Here's how the part is built. I have some questions about the finished solid (model axes, mm). Face numbers are marked on the shaded views. A direction names the side the tool comes from. Coordinates: 2 decimals unless noted, no trailing zeros. Write each loop counter-clockwise with the first axis right and the second up, starting at its lowest first coordinate (ties: lowest second). Pieces come first, ordered by that corner, then holes.
Item 1: I want a section at A-A (y = 6.1). Please give me the cut outline in (x, z) (3 decimals), and give its area (3 significant figures).
Item 2: For the marked faces 1 and 2, which set-ups out of +Z, -Z, +X, -X, +Y, -Y let a thin tool reach every point of the face, with its end or its side?
Item 3: If we mould it in two halves opening along Y, with no side actions, what happens to the marked faces 3, 4, 5 and 6? For each: pulls with the +Y half, pulls with the -Y half, needs draft (parallel to the pull), parting line crosses it, or undercut.
Item 4: I want a section at C-C (x = 3.5). Please give me the cut outline in (y, z) (3 decimals).
Item 5: I want a section at B-B (z = 8.75). Please give me the cut outline in (x, y) (3 decimals).
Item 6: I'm going to push flat-ended pins straight in: P1, Ø1.5, axis at x = 4.5, z = 7, coming from the -Y side; P2, Ø1.1, axis at y = 6, z = 8.5, coming from the -X side; P3, Ø1.1, axis at y = 7, z = 7, coming from the +X side. Where does each tip first touch, or does it pass through?
Item 7: I want a section at D-D (y = 10.5). Please give me the cut outline in (x, z), and give its area (3 significant figures).
Item 8: Please list where these lines run through material, in increasing order: line 1 (Z direction, x = 7, y = 10.25); line 2 (Y direction, x = 4.75, z = 6.25) (3 decimals); line 3 (Y direction, x = 0.75, z = 1.25).
Autodesk Inventor part; units mm, degrees
ref_plane "Work Plane1" through (0, 0, 5) normal (0, 0, 1) x (1, 0, 0)
ref_plane "YZ Plane" through (0, 0, 0) normal (1, 0, 0) x (0, 1, 0)
ref_plane "XZ Plane" through (0, 0, 0) normal (0, 1, 0) x (-1, 0, 0)
sketch "Sketch1" plane through (0, 0, 0) normal (0, 0, 1) x (1, 0, 0)
  line L0 (14.6962, 12.74) -> (14.6962, 0) construction
  line L1 (10.61, 12.2) -> (1.53, 12.2)
  arc A0 (1.53, 12.2) -> (0, 10.67) centre (1.53, 10.67) ccw
  line L2 (0, 10.67) -> (0, 1.53)
  arc A1 (0, 1.53) -> (1.53, 0) centre (1.53, 1.53) ccw
  line L3 (1.53, 0) -> (10.61, 0)
  arc A2 (10.61, 0) -> (12.14, 1.53) centre (10.61, 1.53) ccw
  arc A3 (12.14, 10.67) -> (10.61, 12.2) centre (10.61, 10.67) ccw
  line L4 (12.14, 10.67) -> (12.14, 1.53)
  point P0 (0, 0)
  point P1 (0, 0)
  dimension "d10" = 12.74
ref_plane "Work Plane1" through (0, 0, 5) normal (0, 0, 1) x (1, 0, 0)
sketch "Sketch2" plane through (0, 0, 5) normal (0, 0, 1) x (1, 0, 0)
  line L0 (10.88, 12.74) -> (1.8, 12.74)
  line L1 (10.88, 12.74) -> (1.8, 12.74)
  arc A0 (1.8, 12.74) -> (0, 10.94) centre (1.8, 10.94) ccw
  line L2 (0, 10.94) -> (0, 1.8)
  arc A1 (0, 1.8) -> (1.8, 0) centre (1.8, 1.8) ccw
  line L3 (1.8, 0) -> (10.88, 0)
  arc A2 (10.88, 0) -> (12.68, 1.8) centre (10.88, 1.8) ccw
  line L4 (12.68, 1.8) -> (12.68, 10.94)
  arc A3 (12.68, 10.94) -> (10.88, 12.74) centre (10.88, 10.94) ccw
  circle A4 centre (6.34, 6.37) radius 2.8
  line L5 (5.665, 8.395) -> (7.015, 8.395)
  line L6 (7.015, 4.345) -> (5.665, 4.345)
  line L7 (5.665, 4.345) -> (7.015, 8.395) construction
  line L8 (5.665, 8.395) -> (7.015, 4.345) construction
  line L9 (8.365, 5.695) -> (8.365, 7.045)
  line L10 (4.315, 7.045) -> (4.315, 5.695)
  line L11 (4.315, 5.695) -> (8.365, 7.045) construction
  line L12 (8.365, 5.695) -> (4.315, 7.045) construction
  line L13 (4.315, 5.695) -> (5.665, 5.695)
  line L14 (7.015, 5.695) -> (8.365, 5.695)
  line L15 (5.665, 4.345) -> (5.665, 5.695)
  line L16 (5.665, 7.045) -> (5.665, 8.395)
  line L17 (8.365, 7.045) -> (7.015, 7.045)
  line L18 (5.665, 7.045) -> (4.315, 7.045)
  line L19 (7.015, 8.395) -> (7.015, 7.045)
  line L20 (7.015, 5.695) -> (7.015, 4.345)
  point P0 (0, 0)
  dimension "d3" = 5.6
  dimension "d4" = 4.05
  dimension "d5" = 1.35
  dimension "d6" = 4.05
  dimension "d7" = 1.35
extrude "Extrusion3" add sketch "Sketch1" along normal blind 5
sketch "Sketch3" plane through (0, 0, 5) normal (0, 0, 1) x (1, 0, 0)
  line L0 (10.61, 12.47) -> (1.53, 12.47)
  line L1 (10.61, 12.47) -> (1.53, 12.47)
  arc A0 (1.53, 12.47) -> (-0.27, 10.67) centre (1.53, 10.67) ccw
  line L2 (-0.27, 10.67) -> (-0.27, 1.53)
  arc A1 (-0.27, 1.53) -> (1.53, -0.27) centre (1.53, 1.53) ccw
  line L3 (1.53, -0.27) -> (10.61, -0.27)
  arc A2 (10.61, -0.27) -> (12.41, 1.53) centre (10.61, 1.53) ccw
  line L4 (12.41, 1.53) -> (12.41, 10.67)
  arc A3 (12.41, 10.67) -> (10.61, 12.47) centre (10.61, 10.67) ccw
  circle A4 centre (6.07, 6.1) radius 2.8
  line L5 (5.395, 8.125) -> (6.745, 8.125)
  line L6 (6.745, 4.075) -> (5.395, 4.075)
  line L7 (5.395, 4.075) -> (6.745, 8.125) construction
  line L8 (5.395, 8.125) -> (6.745, 4.075) construction
  line L9 (8.095, 5.425) -> (8.095, 6.775)
  line L10 (4.045, 6.775) -> (4.045, 5.425)
  line L11 (4.045, 5.425) -> (8.095, 6.775) construction
  line L12 (8.095, 5.425) -> (4.045, 6.775) construction
  line L13 (4.045, 5.425) -> (5.395, 5.425)
  line L14 (6.745, 5.425) -> (8.095, 5.425)
  line L15 (5.395, 4.075) -> (5.395, 5.425)
  line L16 (5.395, 6.775) -> (5.395, 8.125)
  line L17 (8.095, 6.775) -> (6.745, 6.775)
  line L18 (5.395, 6.775) -> (4.045, 6.775)
  line L19 (6.745, 8.125) -> (6.745, 6.775)
  line L20 (6.745, 5.425) -> (6.745, 4.075)
  line L21 (10.61, 12.2) -> (1.53, 12.2)
  line L22 (0, 10.67) -> (0, 1.53)
  point P0 (0, 0)
  point P1 (-0.27, -0.27)
  point P2 (6.07, 12.2)
  point P3 (0, 6.1)
  point P4 (6.07, 6.1)
  dimension "d14" = 5.6
  dimension "d15" = 4.05
  dimension "d16" = 1.35
  dimension "d17" = 4.05
  dimension "d18" = 1.35
extrude "Extrusion4" add sketch "Sketch3" along normal blind 4.8 contours A4
sketch "Sketch4" plane through (0, 0, 0) normal (0, 0, -1) x (-1, 0, 0)
  line L0 (-13.9436, 0) -> (-13.9436, 2.266)
  line L1 (-15.5559, 0) -> (-15.5559, 6.84)
  line L2 (-1.53, 0) -> (-10.61, 0)
  line L3 (-11.9098, 9.6363) -> (-0.2302, 9.6363) construction
  line L4 (-0.2302, 9.6363) -> (-0.2302, 6.84) construction
  line L5 (-0.2302, 6.84) -> (-11.9098, 6.84) construction
  line L6 (-11.9098, 6.84) -> (-11.9098, 9.6363) construction
  line L7 (-7.4059, 5.4421) -> (-4.7341, 5.4421) construction
  line L8 (-4.7341, 5.4421) -> (-4.7341, 2.266) construction
  line L9 (-4.7341, 2.266) -> (-7.4059, 2.266) construction
  line L10 (-7.4059, 2.266) -> (-7.4059, 5.4421) construction
  line L11 (-8.8728, 6.8881) -> (-9.5467, 6.8881)
  line L12 (-9.5467, 6.8881) -> (-9.5467, 8.6779)
  line L13 (-9.5467, 8.6779) -> (-10.0369, 7.5227)
  line L14 (-10.0369, 7.5227) -> (-10.5007, 7.5227)
  line L15 (-10.5007, 7.5227) -> (-10.9908, 8.6779)
  line L16 (-10.9908, 8.6779) -> (-10.9908, 6.8881)
  line L17 (-10.9908, 6.8881) -> (-11.6297, 6.8881)
  line L18 (-11.6297, 6.8881) -> (-11.6297, 9.5881)
  line L19 (-11.6297, 9.5881) -> (-10.8486, 9.5881)
  line L20 (-10.8486, 9.5881) -> (-10.2491, 8.2556)
  line L21 (-10.2491, 8.2556) -> (-9.654, 9.5881)
  line L22 (-9.654, 9.5881) -> (-8.8728, 9.5881)
  line L23 (-8.8728, 9.5881) -> (-8.8728, 6.8881)
  line L24 (-7.1924, 7.829) -> (-8.3937, 7.829)
  line L25 (-8.3937, 7.829) -> (-8.3937, 8.3322)
  line L26 (-8.3937, 8.3322) -> (-7.1924, 8.3322)
  line L27 (-7.1924, 8.3322) -> (-7.1924, 7.829)
  spline S0 degree 2 poles (-5.8775, 6.84) (-6.1882, 6.84) (-6.6564, 6.9603) (-6.8577, 7.0479) knots 0 0 0 1 2 2 2
  line L28 (-6.8577, 7.0479) -> (-6.8577, 7.6911)
  line L29 (-6.8577, 7.6911) -> (-6.7964, 7.6911)
  spline S1 degree 2 poles (-6.7964, 7.6911) (-6.5929, 7.5183) (-6.105, 7.3323) (-5.8753, 7.3323) knots 0 0 0 1 2 2 2
  spline S2 degree 2 poles (-5.8753, 7.3323) (-5.8162, 7.3323) (-5.6258, 7.3586) (-5.5689, 7.3848) knots 0 0 0 1 2 2 2
  spline S3 degree 2 poles (-5.5689, 7.3848) (-5.4989, 7.4154) (-5.4005, 7.527) (-5.4005, 7.6167) knots 0 0 0 1 2 2 2
  spline S4 degree 2 poles (-5.4005, 7.6167) (-5.4005, 7.7196) (-5.5602, 7.8465) (-5.6696, 7.8749) knots 0 0 0 1 2 2 2
  spline S5 degree 2 poles (-5.6696, 7.8749) (-5.8074, 7.9121) (-6.1203, 7.9756) (-6.2582, 8.0237) knots 0 0 0 1 2 2 2
  spline S6 degree 2 poles (-6.2582, 8.0237) (-6.5711, 8.1331) (-6.8424, 8.5073) (-6.8424, 8.7873) knots 0 0 0 1 2 2 2
  spline S7 degree 2 poles (-6.8424, 8.7873) (-6.8424, 9.1659) (-6.2013, 9.6363) (-5.7199, 9.6363) knots 0 0 0 1 2 2 2
  spline S8 degree 2 poles (-5.7199, 9.6363) (-5.4792, 9.6363) (-5.0023, 9.5378) (-4.8141, 9.4547) knots 0 0 0 1 2 2 2
  line L30 (-4.8141, 9.4547) -> (-4.8141, 8.8377)
  line L31 (-4.8141, 8.8377) -> (-4.8732, 8.8377)
  spline S9 degree 2 poles (-4.8732, 8.8377) (-5.0241, 8.9667) (-5.4574, 9.144) (-5.6849, 9.144) knots 0 0 0 1 2 2 2
  spline S10 degree 2 poles (-5.6849, 9.144) (-5.7746, 9.144) (-5.9147, 9.1177) (-5.9934, 9.0827) knots 0 0 0 1 2 2 2
  spline S11 degree 2 poles (-5.9934, 9.0827) (-6.0569, 9.0543) (-6.1488, 8.9405) (-6.1488, 8.8705) knots 0 0 0 1 2 2 2
  spline S12 degree 2 poles (-6.1488, 8.8705) (-6.1488, 8.7654) (-6.0022, 8.6451) (-5.7921, 8.597) knots 0 0 0 1 2 2 2
  spline S13 degree 2 poles (-5.7921, 8.597) (-5.6565, 8.5663) (-5.4048, 8.5073) (-5.2604, 8.4569) knots 0 0 0 1 2 2 2
  spline S14 degree 2 poles (-5.2604, 8.4569) (-4.9804, 8.3541) (-4.7069, 8.0128) (-4.7069, 7.7327) knots 0 0 0 1 2 2 2
  spline S15 degree 2 poles (-4.7069, 7.7327) (-4.7069, 7.3301) (-5.3392, 6.84) (-5.8775, 6.84) knots 0 0 0 1 2 2 2
  line L32 (-4.359, 6.8881) -> (-4.359, 9.5881)
  line L33 (-4.359, 9.5881) -> (-2.5342, 9.5881)
  line L34 (-2.5342, 9.5881) -> (-2.5342, 9.074)
  line L35 (-2.5342, 9.074) -> (-3.6851, 9.074)
  line L36 (-3.6851, 9.074) -> (-3.6851, 8.5992)
  line L37 (-3.6851, 8.5992) -> (-2.6239, 8.5992)
  line L38 (-2.6239, 8.5992) -> (-2.6239, 8.085)
  line L39 (-2.6239, 8.085) -> (-3.6851, 8.085)
  line L40 (-3.6851, 8.085) -> (-3.6851, 7.4023)
  line L41 (-3.6851, 7.4023) -> (-2.5342, 7.4023)
  line L42 (-2.5342, 7.4023) -> (-2.5342, 6.8881)
  line L43 (-2.5342, 6.8881) -> (-4.359, 6.8881)
  line L44 (-0.274, 6.8881) -> (-2.0747, 6.8881)
  line L45 (-2.0747, 6.8881) -> (-2.0747, 9.5881)
  line L46 (-2.0747, 9.5881) -> (-1.3964, 9.5881)
  line L47 (-1.3964, 9.5881) -> (-1.3964, 7.4023)
  line L48 (-1.3964, 7.4023) -> (-0.274, 7.4023)
  line L49 (-0.274, 7.4023) -> (-0.274, 6.8881)
  spline S16 degree 2 poles (-4.8947, 3.8553) (-4.8947, 3.4598) (-5.0208, 2.8666) (-5.1617, 2.6664) knots 0 0 0 1 2 2 2
  spline S17 degree 2 poles (-5.1617, 2.6664) (-5.3001, 2.4687) (-5.7475, 2.266) (-6.0688, 2.266) knots 0 0 0 1 2 2 2
  spline S18 degree 2 poles (-6.0688, 2.266) (-6.3925, 2.266) (-6.8374, 2.4687) (-6.9783, 2.6713) knots 0 0 0 1 2 2 2
  spline S19 degree 2 poles (-6.9783, 2.6713) (-7.1192, 2.8716) (-7.2453, 3.4598) (-7.2453, 3.8553) knots 0 0 0 1 2 2 2
  spline S20 degree 2 poles (-7.2453, 3.8553) (-7.2453, 4.2606) (-7.1192, 4.834) (-6.9759, 5.0416) knots 0 0 0 1 2 2 2
  spline S21 degree 2 poles (-6.9759, 5.0416) (-6.8325, 5.2443) (-6.3802, 5.4421) (-6.0688, 5.4421) knots 0 0 0 1 2 2 2
  spline S22 degree 2 poles (-6.0688, 5.4421) (-5.74, 5.4421) (-5.3001, 5.2344) (-5.1592, 5.0293) knots 0 0 0 1 2 2 2
  spline S23 degree 2 poles (-5.1592, 5.0293) (-5.0208, 4.8291) (-4.8947, 4.2384) (-4.8947, 3.8553) knots 0 0 0 1 2 2 2
  spline S24 degree 2 poles (-5.6634, 3.8553) (-5.6634, 4.4213) (-5.8488, 4.8785) (-6.0688, 4.8785) knots 0 0 0 1 2 2 2
  spline S25 degree 2 poles (-6.0688, 4.8785) (-6.2887, 4.8785) (-6.4766, 4.4213) (-6.4766, 3.8528) knots 0 0 0 1 2 2 2
  spline S26 degree 2 poles (-6.4766, 3.8528) (-6.4766, 3.2942) (-6.2887, 2.8295) (-6.0688, 2.8295) knots 0 0 0 1 2 2 2
  spline S27 degree 2 poles (-6.0688, 2.8295) (-5.8513, 2.8295) (-5.6634, 3.2942) (-5.6634, 3.8553) knots 0 0 0 1 2 2 2
  point P0 (0, 0)
  point P1 (-6.07, 0)
  point P2 (-6.07, 2.266)
  point P3 (-6.07, 6.84)
  point P4 (-6.07, 6.84)
  point P5 (-6.07, 2.266)
  dimension "d21" = 2.266
  dimension "d22" = 6.84
extrude "Extrusion5" add sketch "Sketch4" along normal blind 0.9
properties part number "IPC M-SEL 0 key"
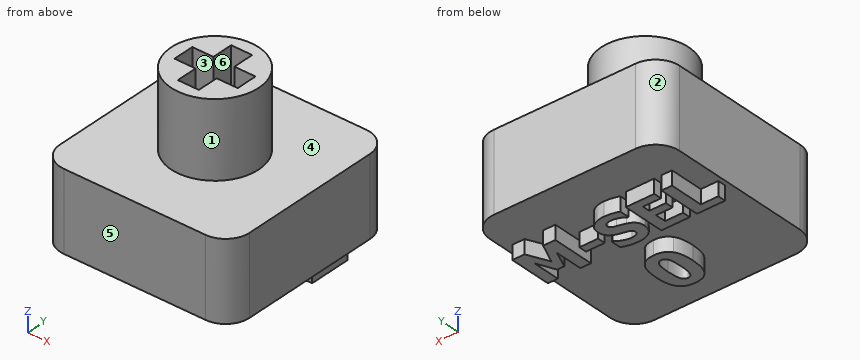
Answer:
1. outline: (0, 0) - (12.14, 0) - (12.14, 5) - (8.87, 5) - (8.87, 9.8) - (8.095, 9.8) - (8.095, 5) - (4.045, 5) - (4.045, 9.8) - (3.27, 9.8) - (3.27, 5) - (0, 5) - close
1. area: 68.1 mm2
2. face 1: +Z
2. face 2: +Z, -Z, -X, +Y
3. face 3: undercut
3. face 4: needs draft
3. face 5: pulls with the -Y half
3. face 6: undercut
4. outline: (0, 0) - (6.888, 0) - (6.888, -0.9) - (7.402, -0.9) - (7.402, 0) - (8.085, 0) - (8.085, -0.9) - (8.599, -0.9) - (8.599, 0) - (9.074, 0) - (9.074, -0.9) - (9.588, -0.9) - (9.588, 0) - (12.2, 0) - (12.2, 5) - (7.211, 5) - (7.211, 9.8) - (4.989, 9.8) - (4.989, 5) - (0, 5) - close
5. outline: circle Ø5.6 at (6.07, 6.1); hole (4.045, 5.425) - (5.395, 5.425) - (5.395, 4.075) - (6.745, 4.075) - (6.745, 5.425) - (8.095, 5.425) - (8.095, 6.775) - (6.745, 6.775) - (6.745, 8.125) - (5.395, 8.125) - (5.395, 6.775) - (4.045, 6.775) - close
6. P1: stops at y = 3.42
6. P2: stops at x = 3.27
6. P3: stops at x = 8.85
7. outline: (0, 0) - (12.14, 0) - (12.14, 5) - (0, 5) - close
7. area: 60.7 mm2
8. line 1: z = 0 to 5
8. line 2: y = 3.631 to 5.425, 6.775 to 8.569
8. line 3: y = 0.21 to 11.99
